Check sheet for the modelled part. Datum: model origin and axes. Units: mm. A direction names the side the tool comes from. Coordinates: 2 decimals unless noted, no trailing zeros. Loops run counter-clockwise (first coordinate to the right, second up) from the corner with the lowest first, then second, coordinate; pieces in that order, holes last. Notation, with made-up numbers: (-33, 88) -> (-2, 88) arc R14 cw to (-2, 108) -> close; hole circle Ø10 at (47.25, -32.75). An arc over 180 degrees is marked (long way). Use CSV: the item, a comma, the result in double quotes.
Autodesk Inventor part; units mm, degrees
ref_plane "YZ Plane" through (0, 0, 0) normal (1, 0, 0) x (0, 1, 0)
ref_plane "XZ Plane" through (0, 0, 0) normal (0, 1, 0) x (-1, 0, 0)
ref_plane "XY Plane" through (0, 0, 0) normal (0, 0, 1) x (1, 0, 0)
sketch "Sketch1" plane through (0, 0, 0) normal (0, 0, 1) x (1, 0, 0)
  circle A0 centre (0, 0) radius 2.9845
  circle A1 centre (0, 0) radius 8.382
  circle A2 centre (0, 0) radius 3.302
  dimension "d0" = 5.969
  dimension "d2" = 0.3175
  dimension "d5" = 5.08
extrude "Extrusion1" add sketch "Sketch1" along normal blind 25.4 contours A1
sketch "Sketch2" plane through (0, 0, 25.4) normal (0, 0, 1) x (1, 0, 0)
  circle A0 centre (0, 0) radius 8.382
extrude "Extrusion2" add sketch "Sketch2" along normal blind 3.175
sketch "Sketch3" plane through (0, 0, 28.575) normal (0, 0, 1) x (1, 0, 0)
  line L0 (0.635, -2.54) -> (-0.635, -2.54)
  line L1 (-0.635, -2.54) -> (-0.635, 2.54)
  line L2 (-0.635, 2.54) -> (0.635, 2.54)
  line L3 (0.635, 2.54) -> (0.635, -2.54)
  line L4 (0.635, -2.54) -> (-0.635, 2.54) construction
  line L5 (-0.635, -2.54) -> (0.635, 2.54) construction
  line L6 (0, 2.54) -> (0, -2.54) construction
  line L7 (-1.905, -2.54) -> (1.905, -2.54)
  line L8 (1.905, -2.54) -> (0, -5.9267)
  line L9 (0, -5.9267) -> (-1.905, -2.54)
  point P0 (0, 0)
  dimension "d8" = 5.08
  dimension "d10" = 1.27
  dimension "d11" = 3.81
  dimension "d45" = 3.3867
extrude "Extrusion3" cut sketch "Sketch3" against normal blind 1.27
chamfer "Chamfer1" distance 0.508 angle 45 1 edges at (-8.382, 0, 28.575)
sketch "Sketch6" plane through (0, 0, 25.4) normal (0, 0, -1) x (-1, 0, 0)
  circle A0 centre (0, 0) radius 3.302
  line L0 (0.6206, 3.2432) -> (3.1189, -1.0842)
  line L1 (3.1189, 1.0842) -> (0.6206, -3.2432) construction
  line L2 (0, 0) -> (3.302, 0) construction
  circle A1 centre (0, 0) radius 3.302 construction
  line L3 (0, 0) -> (2.8596, -1.651) construction
  line L4 (0, 0) -> (2.8596, 1.651) construction
  line L5 (-1.3144, 4.3273) -> (-3.8128, 0) construction
  arc A2 (0.6206, -3.2432) -> (3.1189, 1.0842) centre (0, 0) ccw
  arc A3 (3.1189, -1.0842) -> (0.6206, 3.2432) centre (0, 0) ccw
  circle A4 centre (0, 0) radius 3.302
  dimension "d24" = 60
  dimension "d26" = 5.461
extrude "Extrusion6" add sketch "Sketch6" along normal blind 10.16 contours A0 L0 picked at (2.0493, 1.4727)
sketch "Sketch10" plane through (0, 0, 0) normal (0, 0, -1) x (-1, 0, 0)
  circle A0 centre (0, 0) radius 6.35
  circle A1 centre (0, 0) radius 11.43
  circle A2 centre (0, 0) radius 3.302 construction
  circle A3 centre (0, 0) radius 8.382 construction
  dimension "d49" = 12.7
  dimension "d50" = 5.08
  dimension "d51" = 5.08
extrude "Extrusion10" add sketch "Sketch10" against normal blind 2.54
chamfer "Chamfer3" distance 6.35 distance2 3.048 1 edges at (-8.382, 0, 2.54) measured on face at (8.2735, 1.3446, 11.049)
sketch "Sketch11" plane through (0, 0, 0) normal (0, 0, -1) x (-1, 0, 0)
  circle A0 centre (0, 0) radius 6.35
  dimension "d57" = 12.7
extrude "Extrusion11" cut sketch "Sketch11" against normal blind 5.08
chamfer "Chamfer4" distance 3.048 angle 45 1 edges at (6.35, 0, 5.08)
equation "\"d11\" = 3 * d10"
equation "\"d45\" = 0.666667 * d8"
equation "\"d51\" = d50"
properties part number "potcap"
1) Go/stop test with flat-tipped pins: pin 1 Ø0.6 at (y, z) = (1, 27.5) entering from +X; pin 2 Ø1.4 at (x, z) = (1, 28) entering from -Y; pin 3 Ø3.5 at (x, y) = (-1, -0.5) entering from -Z. Record where each tip stops, or that it passes through.
Answer below:
pin 1,"stops at x = 8.35"
pin 2,"stops at y = -8.38"
pin 3,"stops at z = 15.24"
2) Draft check along Y on faces 1 (the conical face through (7.92, 3.28, 8.49)), 2 (the flat face through (-2, 2, 15.24)), 3 (the flat face through (-5, -5, 0)). Enter one of: released by +Y, released by -Y, zero draft, split by the parting line, or undercut.
Answer below:
face 1,"split by the parting line"
face 2,"undercut"
face 3,"zero draft"
3) Access from +Z, -Z, +X, -X, +Y, -Y to the whole of each face (thin tool, end or side, straight path). Record for faces 4 (the cylindrical face through (1.38, -6.2, 1)), 5 (the flat face through (-0.635, 0, 28)), 6 (the flat face through (2, 0, 28.575)).
Answer below:
face 4,"-Z"
face 5,"+Z"
face 6,"+Z, +X, -X, +Y, -Y"
4) Thickness scan on line 1 along Y through (x, z) = (0, 0.75); line 2 along Y through (x, z) = (0, 10.75); line 3 along Z through (x, y) = (0.5, 0.25) (3 decimals). Record the ranges inside material, lowest first. Write a range as from..to.
Answer below:
line 1,"y = -11.43..-6.35, 6.35..11.43"
line 2,"y = -8.38..-3.3, 3.3..8.38"
line 3,"z = 25.4..27.305"
5) Cross-section at C-C on z = 8.5. Record the boundary of the cut face in (x, y).
Answer below:
outline,"circle Ø17.14 at (0, 0); hole circle Ø6.6 at (0, 0)"
6) Cross-section at B-B on z = 25. Record the boundary of the cut face in (x, y), and give its area (3 significant figures).
Answer below:
outline,"circle Ø16.76 at (0, 0); hole (-3.12, -1.08) arc R3.3 ccw (long way) to (-0.62, 3.24) -> close"
area,"190 mm²"
